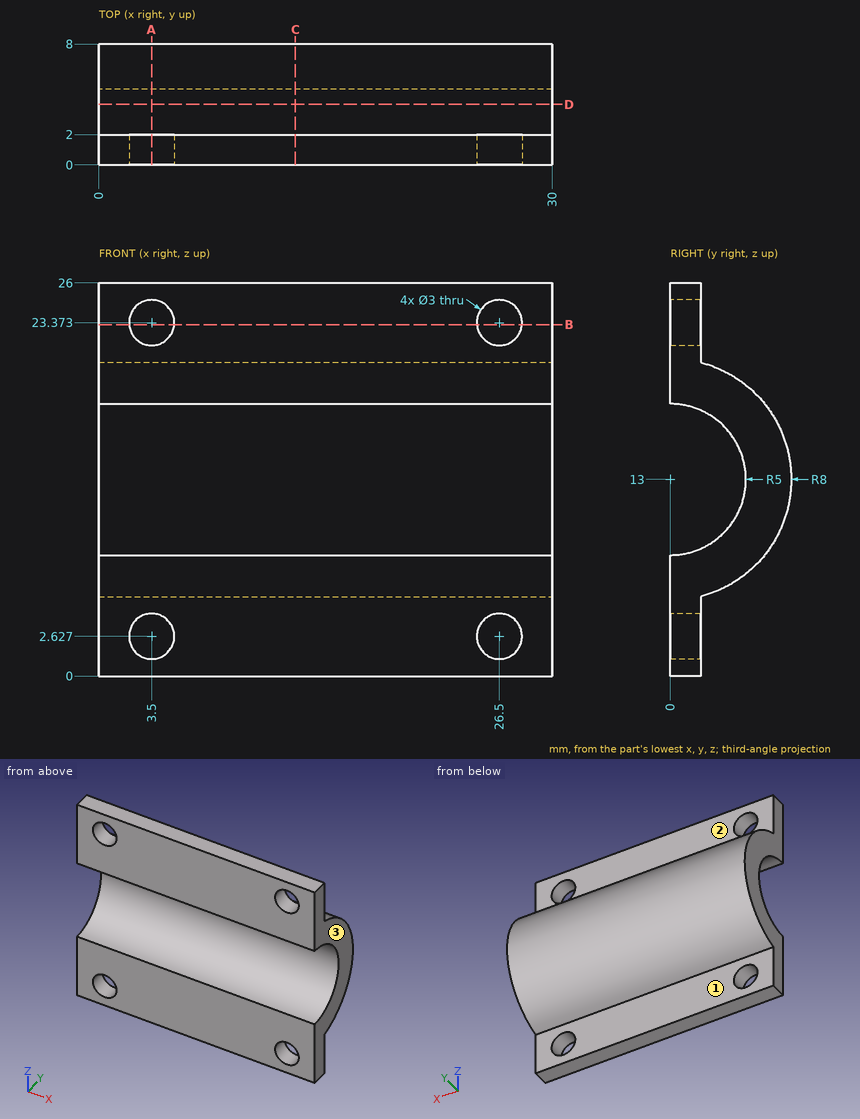
Here's the drawing with two shaded views (mm, measured from the low corner). I have some questions. A direction names the side the tool comes from. Round coordinates to 2 decimals unless told otherwise and drop trailing zeros. Order: outer loops, then holes, each group sorted by start corner. A loop starts at its lowest first (then second) coordinate and runs counter-clockwise, first axis right, second up. Notation, with made-up numbers: M 72,29.25 L 106,29.25 A26 ccw 106,68.25 Z; hole C 66.25,45.25 d8. An arc over 180 degrees is marked long. Use CSV: the item, a comma, the result in double quotes.
1) On a 3-axis mill with a long thin cutter (end or side, diameter ignored), from which of +Z, -Z, +X, -X, +Y, -Y can I reach the whole of each face in a straight line? I mean the marked faces 1, 2 and 3. Say none if no direction works.
Taken from the geometry:
face 1,"-Z, +X, -X, +Y"
face 2,"+Z, +X, -X, +Y"
face 3,"+Z, -Z, +X, +Y, -Y"
2) I need wall thicknesses on line 1 along Z through (x, y) = (17.25, 3.5); line 2 along Z through (x, y) = (23.75, 2.25); line 3 along Y through (x, z) = (7.5, 21.5). Which ranges of each line are inside material? Lowest first, please. Write a range as [from, to].
Taken from the geometry:
line 1,"[5.81, 9.43], [16.57, 20.19]"
line 2,"[5.32, 8.53], [17.47, 20.68]"
line 3,"[0, 2]"
3) I want a section at D-D (y = 4). List the corners of the cut face in (x, z) for me.
Taken from the geometry:
outline,"M 0,6.07 L 30,6.07 L 30,10 L 0,10 Z; M 0,16 L 30,16 L 30,19.93 L 0,19.93 Z"
4) I'm going to push flat-ended pins straight in: P1, Ø5, axis at x = 19, z = 10, coming from the +Y side; P2, Ø1.6, axis at x = 19, z = 2, coming from the +Y side; P3, Ø2, axis at x = 24, z = 17.5, coming from the -Y side; P4, Ø8, axis at x = 11, z = 4, coming from the +Y side (3 decimals). Where does each tip first touch, or does it pass through?
Taken from the geometry:
P1,"y = 7.98"
P2,"y = 2"
P3,"y = 0"
P4,"y = 6.245"
5) I want a section at C-C (x = 13). List the corners of the cut face in (y, z) for me.
Taken from the geometry:
outline,"M 0,0 L 2,0 L 2,5.25 A8 ccw 2,20.75 L 2,26 L 0,26 L 0,18 A5 cw 0,8 Z"
6) I want a section at A-A (x = 3.5). List the corners of the cut face in (y, z) for me, then the cut area to 3 significant figures.
Taken from the geometry:
outline,"M 0,0 L 2,0 L 2,1.13 L 0,1.13 Z; M 0,4.13 L 2,4.13 L 2,5.25 A8 ccw 2,20.75 L 2,21.87 L 0,21.87 L 0,18 A5 cw 0,8 Z; M 0,24.87 L 2,24.87 L 2,26 L 0,26 Z"
area,"69.6 mm^2"
7) I want a section at B-B (z = 23.25). List the corners of the cut face in (x, y) for me, then the cut area to 3 significant figures.
Taken from the geometry:
outline,"M 0,0 L 2.01,0 L 2.01,2 L 0,2 Z; M 4.99,0 L 25.01,0 L 25.01,2 L 4.99,2 Z; M 27.99,0 L 30,0 L 30,2 L 27.99,2 Z"
area,"48.0 mm^2"
